Source: CAD feature listing. Evaluate the final solid. Frame: model axes, mm. A direction names the side the tool comes from. Coordinates: 2 decimals unless noted, no trailing zeros. Write each loop counter-clockwise with the first axis right and the second up, starting at its lowest first coordinate (ties: lowest second). Pieces come first, ordered by that corner, then holes. Notation, with made-up numbers: (5.25, 54.5) - (41.25, 54.5) arc R10 cw to (41.25, 73.5) - close; hole circle Ø10 at (30, 27.5). An arc over 180 degrees is marked (long way). One line per question, with ' | ' between items.
from build123d import *

# Parameters (mm, degrees)
F0_R     = 23
F0_R_2   = 18.5
F1_DEPTH = 2.2
F2_R     = 28.7689848305
F2_R_2   = 21.0167623051
F3_DEPTH = 6.35
F5_DEPTH = 6.35
F8_W     = 86.7
F8_H     = 75.3333002466
F9_DEPTH = 6.35


with BuildPart() as f1:
    # F0 (on Right) → F1 (new body)
    with BuildSketch(Plane.YZ):
        Circle(F0_R)
        Circle(F0_R_2, mode=Mode.SUBTRACT)
    extrude(amount=F1_DEPTH)

    # F2 (on Right) → F3 (join)
    with BuildSketch(Plane.YZ):
        Circle(F2_R)
        Circle(F2_R_2, mode=Mode.SUBTRACT)
    extrude(amount=F3_DEPTH)

    # F4 (on Right) → F5 (join)
    with BuildSketch(Plane.YZ):
        with BuildLine():
            Line((61.2828924653, 28.7689848305), (0, 28.7689848305))
            ThreePointArc((0, 28.7689848305), (28.652224252, -2.5893114127), (-5.1576050869, -28.3028902754))
            Line((-5.1576050869, -28.3028902754), (61.2828924653, -46.5643154161))
            Line((61.2828924653, -46.5643154161), (61.2828924653, 28.7689848305))
        make_face()
    extrude(amount=F5_DEPTH)


with BuildPart() as f6_1:
    # F6: instance of F1
    add(f1.part.mirror(Plane.YZ))


with BuildPart() as f6_1_1:
    # F7: moved
    add(f6_1.part.moved(Location((-74, 0, 0))))


with BuildPart() as f1_1:
    add(f1.part)

    add(f6_1_1.part)  # F9 merges F6_1
    # F8 (on face) → F9 (join)
    with BuildSketch(Plane(origin=(0, 61.2828924653, 0), x_dir=(-1, 0, 0), z_dir=(0, 1, 0))):
        with Locations((37, -8.8976652928)):
            Rectangle(F8_W, F8_H)
    extrude(amount=F9_DEPTH)


solid = f1_1.part
Item 1: Cut plane B-B on y = -15.5. Return loops of the section in (x, z).
Check sheet entries:
outline: (-80.35, -24.24) - (-74, -24.24) - (-74, -10.1) - (-76.2, -10.1) - (-76.2, -14.19) - (-80.35, -14.19) - close; (-80.35, 14.19) - (-76.2, 14.19) - (-76.2, 10.1) - (-74, 10.1) - (-74, 24.24) - (-80.35, 24.24) - close; (0, -24.24) - (6.35, -24.24) - (6.35, -14.19) - (2.2, -14.19) - (2.2, -10.1) - (0, -10.1) - close; (0, 10.1) - (2.2, 10.1) - (2.2, 14.19) - (6.35, 14.19) - (6.35, 24.24) - (0, 24.24) - close
Item 2: Cut plane A-A on z = 0. Return loops of the section in (x, y), and give its area (3 significant figures).
Check sheet entries:
outline: (-80.35, -28.77) - (-74, -28.77) - (-74, -18.5) - (-76.2, -18.5) - (-76.2, -21.02) - (-80.35, -21.02) - close; (-80.35, 21.02) - (-76.2, 21.02) - (-76.2, 18.5) - (-74, 18.5) - (-74, 61.28) - (0, 61.28) - (0, 18.5) - (2.2, 18.5) - (2.2, 21.02) - (6.35, 21.02) - (6.35, 67.63) - (-80.35, 67.63) - close; (0, -28.77) - (6.35, -28.77) - (6.35, -21.02) - (2.2, -21.02) - (2.2, -18.5) - (0, -18.5) - close | area: 1,180 mm²
Item 3: Cut plane C-C on y = 47.5. Return loops of the section in (x, z).
Check sheet entries:
outline: (-80.35, -42.78) - (-74, -42.78) - (-74, 28.77) - (-80.35, 28.77) - close; (0, -42.78) - (6.35, -42.78) - (6.35, 28.77) - (0, 28.77) - close
Item 4: Access query for faces 1 (the face through (4.246, -4.556, -20.517)), 2 (the face through (-76.2, 0, -19)), 3 (the face through (3.131, -28.592, 3.183)), 4 (the face through (0, 26, -8)), 5 (the face through (1.08, -4.01, -18.06)). Directions: +Z, -Z, +X, -X, +Y, -Y. A direction counts if a zero-diameter tool reaches every point of the face in a straight line with its end or side. Return the directions, or none.
Check sheet entries:
face 1: +X | face 2: -X | face 3: +X, -X, -Y | face 4: +Z, -Z, -Y | face 5: +X, -X
Item 5: Cut plane D-D on x = -51.5. Return loops of the section in (y, z).
Check sheet entries:
outline: (61.28, -46.56) - (67.63, -46.56) - (67.63, 28.77) - (61.28, 28.77) - close
Item 6: Ray query, line 1 along X through (y, z) = (12.5, -33); line 2 along Y through (x, z) = (-77, 0); line 3 along Y through (x, z) = (-43, -25.5). Return the intervals inside material, ascending. Write a range as [from, to].
Check sheet entries:
line 1: [-80.35, -74], [0, 6.35] | line 2: [-28.77, -21.02], [21.02, 67.63] | line 3: [61.28, 67.63]
Item 7: Mould query, pull axis X, two halves, no side actions, for faces 6 (the face through (2.2, 0, -19)), 7 (the face through (-36, 61.283, -8)), 8 (the face through (-78.246, -4.556, -20.517)), 9 (the face through (-74, 26, -8)). Classes: pulls with the +X half, pulls with the -X half, needs draft (parallel to the pull), parting line crosses it, or undercut.
Check sheet entries:
face 6: pulls with the +X half | face 7: undercut | face 8: needs draft | face 9: undercut
